```python
from build123d import *

# Parameters (mm, degrees)
SKETCH1_W           = 250
SKETCH1_H           = 300
BOSS_EXTRUDE1_DEPTH = 100
SKETCH2_W           = 15
SKETCH2_H           = 15
BOSS_EXTRUDE2_DEPTH = 7.5
FILLET1_R           = 7.5
SKETCH3_R           = 7.5
BOSS_EXTRUDE3_DEPTH = 10
BOSS_EXTRUDE4_START = -10
SKETCH4_R           = 7.5
BOSS_EXTRUDE4_DEPTH = 10


with BuildPart() as part:
    # Sketch1 → Boss-Extrude1 (new body)
    with BuildSketch(Plane.XY):
        Rectangle(SKETCH1_W, SKETCH1_H)
    extrude(amount=BOSS_EXTRUDE1_DEPTH)

    # Sketch2 → Boss-Extrude2 (add)
    with BuildSketch(Plane(origin=(0, 0, 0), x_dir=(-1, 0, 0), z_dir=(0, 0, -1))):
        with Locations((0, 100)):
            Rectangle(SKETCH2_W, SKETCH2_H)
        with Locations((0, -100)):
            Rectangle(SKETCH2_W, SKETCH2_H)
    extrude(amount=BOSS_EXTRUDE2_DEPTH)

    # Fillet1
    fillet1_edges = [part.edges().sort_by_distance(p)[0] for p in [
        (0, 107.5, -7.5),
        (0, 92.5, -7.5),
        (0, -107.5, -7.5),
        (0, -92.5, -7.5),
    ]]
    fillet(fillet1_edges, radius=FILLET1_R - 0.0001)  # a hair under: the kernel refuses the full size

    # Sketch3 → Boss-Extrude3 (add)
    with BuildSketch(Plane.ZY.offset(125)):
        with Locations((0, 100)):
            Circle(SKETCH3_R)
        with Locations((0, -100)):
            Circle(SKETCH3_R)
    extrude(amount=-BOSS_EXTRUDE3_DEPTH)

    # Sketch4 → Boss-Extrude4 (add)
    with BuildSketch(Plane(origin=(125, 0, 0), x_dir=(0, 0, -1), z_dir=(1, 0, 0)).offset(BOSS_EXTRUDE4_START)):
        with Locations((0, 100)):
            Circle(SKETCH4_R)
        with Locations((0, -100)):
            Circle(SKETCH4_R)
    extrude(amount=BOSS_EXTRUDE4_DEPTH)


solid = part.part
```
The listing builds one solid part. Answer for the finished solid, in the listing's coordinates (mm). A direction names the side the tool comes from. Coordinates: 2 decimals unless noted, no trailing zeros. Write each loop counter-clockwise with the first axis right and the second up, starting at its lowest first coordinate (ties: lowest second). Pieces come first, ordered by that corner, then holes.
Q1. Which of the six approach directions +Z, -Z, +X, -X, +Y, -Y give full straight-line access (tool end or side, diameter ignored) to faces 1 (the flat face through (-7.5, 100, -3)), 2 (the cylindrical face through (-0.105, 94.639, -5.245)), 3 (the flat face through (-2, 2, 100))?
Returned:
face 1: -Z, +Y, -Y
face 2: -Z, +X, -X
face 3: +Z, +X, -X, +Y, -Y
Q2. Section A-A, the plane x = -35 is taken. Write down the section's boundary in (y, z), then the cut area to 3 significant figures.
Returned:
outline: (-150, 0) - (150, 0) - (150, 100) - (-150, 100) - close
area: 30,000 mm2
Q3. Section B-B, the plane y = 119 is taken. Write down the section's boundary in (x, z).
Returned:
outline: (-125, 0) - (125, 0) - (125, 100) - (-125, 100) - close
Q4. The mould has two halves that part along X. Classify faces 4 (the flat face through (-115, 100, -3)), 5 (the flat face through (-125, -2, 45)), 6 (the flat face through (-2, 150, 49)): released by +X, released by -X, zero draft, split by the parting line, or undercut.
Returned:
face 4: undercut
face 5: released by -X
face 6: zero draft
Q5. Given P1, Ø2, axis at x = 90, y = 0, coming from the -Z side, flat-ended and moving along its own axis, determine where the tip first touches the part or whether it passes through.
Returned:
P1: stops at z = 0
Q6. Find the intervals of material crossed by line 1 along Z through (x, y) = (-98, -78), in increasing order.
Returned:
line 1: z = 0 to 100
